Part print with two shaded views. Sizes in mm from the minimum x, y, z corner. A direction names the side the tool comes from. Round coordinates to 2 decimals unless told otherwise and drop trailing zeros. Write each loop counter-clockwise with the first axis right and the second up, starting at its lowest first coordinate (ties: lowest second). Pieces come first, ordered by that corner, then holes. Notation, with made-up numbers: (88, 11) -> (119, 11) arc R19 ccw to (119, 45) -> close; hole circle Ø6 at (31.25, 20.5). An arc over 180 degrees is marked (long way). Answer in a Markdown table with one row per item.
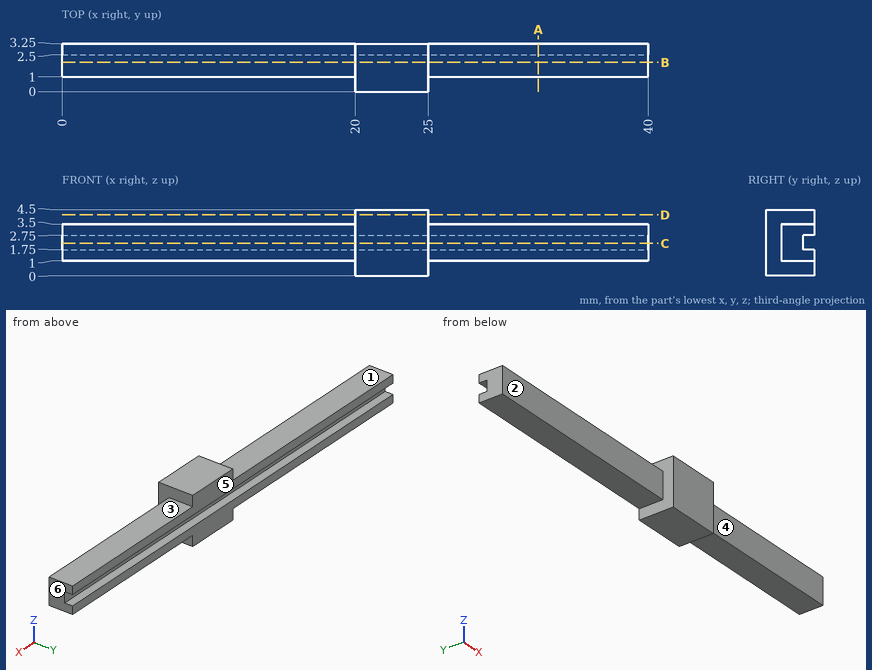
Q1. Saw through at C-C on z = 2.2. Write the cut outline in (x, y), plus the area to 3 significant figures.
A:
| item | result |
|---|---|
| outline | (0, 1) -> (20, 1) -> (20, 0) -> (25, 0) -> (25, 1) -> (40, 1) -> (40, 2.5) -> (0, 2.5) -> close |
| area | 65.0 mm² |
Q2. Wall check: line 1 (Z direction, x = 37, y = 2.55); line 2 (Y direction, x = 18, z = 1.95); line 3 (X direction, y = 0.8, z = 2.9). Give the ranges that are in metal, low to high. Write a range as [from, to].
A:
| item | result |
|---|---|
| line 1 | [1, 1.75], [2.75, 3.5] |
| line 2 | [1, 2.5] |
| line 3 | [20, 25] |
Q3. Saw through at D-D on z = 4.15. Write the cut outline in (x, y).
A:
| item | result |
|---|---|
| outline | (20, 0) -> (25, 0) -> (25, 3.25) -> (20, 3.25) -> close |
Q4. Saw through at A-A on x = 32.5. Write the cut outline in (y, z).
A:
| item | result |
|---|---|
| outline | (1, 1) -> (3.25, 1) -> (3.25, 1.75) -> (2.5, 1.75) -> (2.5, 2.75) -> (3.25, 2.75) -> (3.25, 3.5) -> (1, 3.5) -> close |
Q5. Saw through at B-B on y = 2. Write the cut outline in (x, z), plus the area to 3 significant figures.
A:
| item | result |
|---|---|
| outline | (0, 1) -> (20, 1) -> (20, 0) -> (25, 0) -> (25, 1) -> (40, 1) -> (40, 3.5) -> (25, 3.5) -> (25, 4.5) -> (20, 4.5) -> (20, 3.5) -> (0, 3.5) -> close |
| area | 110 mm² |
Q6. Which spindle directions (+Z, -Z, +X, -X, +Y, -Y) get a long thin tool onto all of the face, cutting with end or side? Do the marked faces 1, 2, 3 and 4. Say none if no direction does.
A:
| item | result |
|---|---|
| face 1 | +Z, -X, +Y, -Y |
| face 2 | +Z, -Z, -X, -Y |
| face 3 | +Z, +X, +Y, -Y |
| face 4 | +Z, -Z, +X, -Y |
Q7. Two-plate mould, pull along X, no slides. Class the marked faces 5 and 6: released by +X, released by -X, zero draft, split by the parting line, or undercut.
A:
| item | result |
|---|---|
| face 5 | zero draft |
| face 6 | released by +X |
Q8. Drop flat-ended pins along their axis: P1, Ø0.7, axis at x = 34, y = 2, coming from the +Z side; P2, Ø0.7, axis at x = 34, y = 2.5, coming from the -Z side; P3, Ø2, axis at x = 32.5, z = 2.5, coming from the -Y side; P4, Ø1.5, axis at y = 1, z = 3, coming from the -X side. Give the stop position or say it passes through.
A:
| item | result |
|---|---|
| P1 | z = 3.5 |
| P2 | z = 1 |
| P3 | y = 1 |
| P4 | x = 0 |
